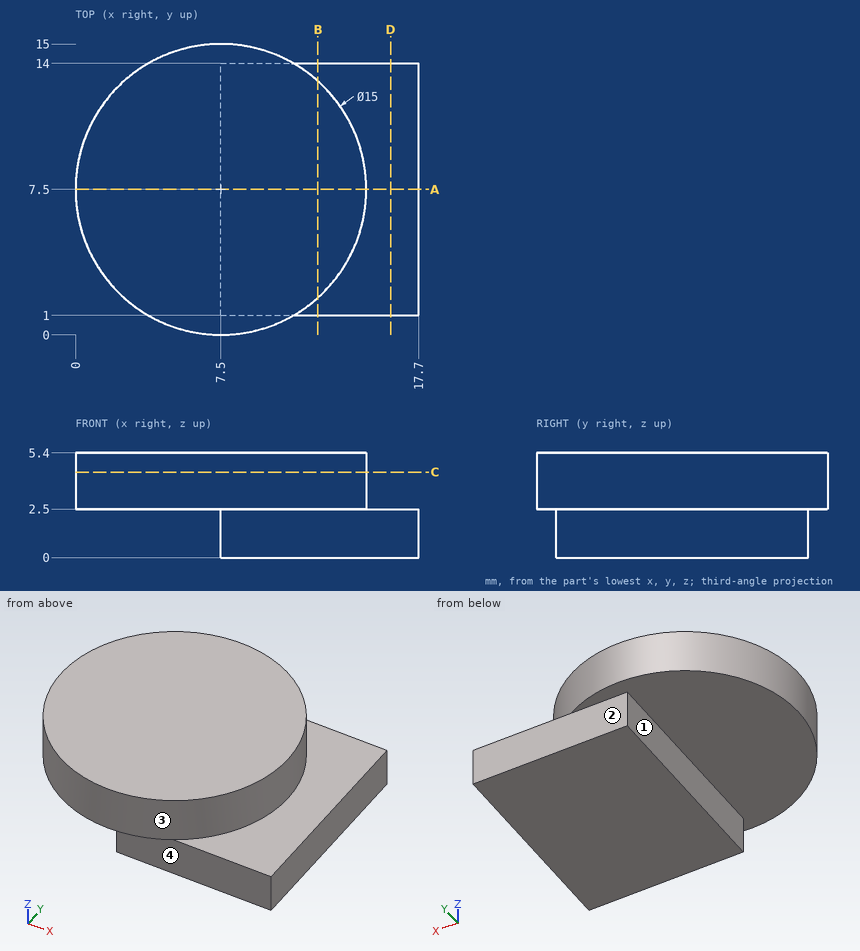
Verification items for this drawing (mm, ordinates from the low corner). A direction names the side the tool comes from. Round coordinates to 2 decimals unless told otherwise and drop trailing zeros. Order: outer loops, then holes, each group sorted by start corner. A loop starts at its lowest first (then second) coordinate and runs counter-clockwise, first axis right, second up. Notation, with made-up numbers: (-2, 20.25) - (36, 20.25) arc R14 cw to (36, 31.25) - close; hole circle Ø6 at (-15, -24.5). An arc over 180 degrees is marked (long way). Use CSV: the item, a comma, the result in double quotes. Start each with the question number.
1) Go/stop test with flat-tipped pins: P1, Ø2, axis at x = 13, z = 1, coming from the -Y side; P2, Ø0.8, axis at x = 13, z = 1.5, coming from the +Y side; P3, Ø3, axis at y = 7.5, z = 1.5, coming from the -X side. Record where each tip stops, or that it passes through.
2) Section check D-D, the plane x = 16.25. Record the cut outline in (y, z).
3) Section check A-A, the plane y = 7.5. Record the cut outline in (x, z), plus the area to 3 significant figures.
4) Section check B-B, the plane x = 12.5. Record the cut outline in (y, z), plus the area to 3 significant figures.
5) Access from +Z, -Z, +X, -X, +Y, -Y to the whole of each face (thin tool, end or side, straight path). Record for the marked faces 1, 2, 3 and 4.
6) Section check C-C, the plane z = 4.4. Record the cut outline in (x, y), plus the area to 3 significant figures.
7) Thickness scan on L1, parallel to X at y = 9.25, z = 1.75; L2, parallel to Z at x = 15.5, y = 7.5; L3, parallel to Z at x = 1.25, y = 3.75. Record the ranges inside material, lowest first.
Answers:
1,P1,"stops at y = 1"
1,P2,"stops at y = 14"
1,P3,"stops at x = 0"
2,outline,"(1, 0) - (14, 0) - (14, 2.5) - (1, 2.5) - close"
3,outline,"(0, 2.5) - (7.5, 2.5) - (7.5, 0) - (17.7, 0) - (17.7, 2.5) - (15, 2.5) - (15, 5.4) - (0, 5.4) - close"
3,area,"69.0 mm²"
4,outline,"(1, 0) - (14, 0) - (14, 2.5) - (13.09, 2.5) - (13.09, 5.4) - (1.91, 5.4) - (1.91, 2.5) - (1, 2.5) - close"
4,area,"64.9 mm²"
5,face 1,"-Z, -X, +Y, -Y"
5,face 2,"-Z, +X, -X, +Y"
5,face 3,"+Z"
5,face 4,"-Z, +X, -X, -Y"
6,outline,"circle Ø15 at (7.5, 7.5)"
6,area,"177 mm²"
7,L1,"x = 7.5 to 17.7"
7,L2,"z = 0 to 2.5"
7,L3,"z = 2.5 to 5.4"
